```python
from build123d import *

# Parameters (mm, degrees)
F0_W      = 180
F0_H      = 40
F1_DEPTH  = 15
F2_W      = 60
F2_H      = 40
F3_DEPTH  = 120
F4_W      = 41
F4_H      = 40
F5_DEPTH  = 115
F6_R      = 20
F7_R      = 5
F8_W      = 30
F8_H      = 20
F9_DEPTH  = 40
F10_W     = 30
F10_H     = 20
F11_DEPTH = 40
F13_D     = 22
F13_DEPTH = 12
F13_TIP   = 6.6094668093
F15_D     = 22
F15_DEPTH = 12
F15_TIP   = 6.6094668093


with BuildPart() as f1:
    # F0 (on Front) → F1 (new body, symmetric)
    with BuildSketch(Plane.XZ):
        with Locations((0, 6.5696623251)):
            Rectangle(F0_W, F0_H)
    extrude(amount=F1_DEPTH, both=True)

    # F2 (on face) → F3 (join)
    with BuildSketch(Plane.XZ.offset(15)):
        with Locations((0, 6.5696623251)):
            Rectangle(F2_W, F2_H)
    extrude(amount=F3_DEPTH)

    # F4 (on face) → F5 (cut)
    with BuildSketch(Plane.XZ.offset(135)):
        with Locations((0, 6.5696623251)):
            Rectangle(F4_W, F4_H)
    extrude(amount=-F5_DEPTH, mode=Mode.SUBTRACT)

    # F6
    f6_edges = [f1.edges().sort_by_distance(p)[0] for p in [
        (-30, -15, 6.569662),
        (30, -15, 6.569662),
    ]]
    fillet(f6_edges, radius=F6_R)

    # F7
    f7_edges = [f1.edges().sort_by_distance(p)[0] for p in [
        (-20.5, -20, 6.569662),
        (20.5, -20, 6.569662),
        (-20.5, -135, 6.569662),
        (20.5, -135, 6.569662),
    ]]
    fillet(f7_edges, radius=F7_R)

    # F8 (on face) → F9 (cut)
    with BuildSketch(Plane.XY.offset(26.5696623251)):
        with Locations((-70, 0)):
            Rectangle(F8_W, F8_H)
    extrude(amount=-F9_DEPTH, mode=Mode.SUBTRACT)

    # F10 (on face) → F11 (cut)
    with BuildSketch(Plane.XY.offset(26.5696623251)):
        with Locations((70, 0)):
            Rectangle(F10_W, F10_H)
    extrude(amount=-F11_DEPTH, mode=Mode.SUBTRACT)

    # F13
    with Locations(Plane.XZ.offset(15)):
        with Locations((-70, 6.5696623251)):
            Hole(F13_D / 2, depth=F13_DEPTH)
            with Locations((0, 0, -(F13_DEPTH + F13_TIP / 2))):  # 118° drill point
                Cone(0, F13_D / 2, F13_TIP, mode=Mode.SUBTRACT)

    # F15
    with Locations(Plane.XZ.offset(15)):
        with Locations((70, 6.5696623251)):
            Hole(F15_D / 2, depth=F15_DEPTH)
            with Locations((0, 0, -(F15_DEPTH + F15_TIP / 2))):  # 118° drill point
                Cone(0, F15_D / 2, F15_TIP, mode=Mode.SUBTRACT)


solid = f1.part
```
Verification items for the finished model (mm, model axes). A direction names the side the tool comes from. Round coordinates to 2 decimals unless told otherwise and drop trailing zeros. Write each loop counter-clockwise with the first axis right and the second up, starting at its lowest first coordinate (ties: lowest second). Pieces come first, ordered by that corner, then holes. Notation, with made-up numbers: (37, -10.75) - (46, -10.75) arc R16 ccw to (46, 1.25) - close; hole circle Ø11 at (-27, 3). An arc over 180 degrees is marked (long way). Answer as a JSON object with one key per item and string values. Group by question number.
Q1. Thickness scan on line 1 (Z direction, x = -70, y = -12); line 2 (X direction, y = -85.5, z = -10); line 3 (Y direction, x = 61.5, z = -4). Record the ranges inside material, lowest first.
Q2. Section check A-A, the plane y = -108. Enter the section's corners in (x, z), plus the area to 3 significant figures.
Q3. Section check D-D, the plane z = 22. Enter the section's corners in (x, y).
Q4. Go/stop test with flat-tipped pins: pin 1 Ø20 at (x, z) = (-80, 5.5) entering from -Y; pin 2 Ø20 at (y, z) = (-80, 13) entering from +X; pin 3 Ø20 at (y, z) = (-82.5, 15.5) entering from -X; pin 4 Ø6 at (x, y) = (58.5, -8.5) entering from +Z. Record where each tip stops, or that it passes through.
Q5. Section check C-C, the plane x = -70. Enter the section's corners in (y, z).
Q6. Section check B-B, the plane y = 5. Enter the section's corners in (x, z), plus the area to 3 significant figures.
Q7. Tool access check on faces 1 (the flat face through (-79, -15, -2)), 2 (the flat face through (30, -84, 6)), 3 (the flat face through (90, 0, 6)), 4 (the flat face through (-70, 10, 7)), 5 (the cylindrical face through (-22, -133.57, 6.85)). Record the directions out of +Z, -Z, +X, -X, +Y, -Y that give a thin tool (end or side, any length) a straight path to the whole face; none if there is none.
Q8. Mould release check, pull along Y, two halves, no side actions. Record for faces 6 (the flat face through (-55, 0, 7)), 7 (the flat face through (0, -20, 7)), 8 (the flat face through (0, -16, -13.43)), 9 (the flat face through (70, 10, 7)): released by +Y, released by -Y, zero draft, split by the parting line, or undercut.
Found:
{
 "1": {"line 1": "z = -13.43 to -4.43, 17.57 to 26.57", "line 2": "x = -30 to -20.5, 20.5 to 30", "line 3": "y = -15 to -10, 10 to 15"},
 "2": {"outline": "(-30, -13.43) - (-20.5, -13.43) - (-20.5, 26.57) - (-30, 26.57) - close; (20.5, -13.43) - (30, -13.43) - (30, 26.57) - (20.5, 26.57) - close", "area": "760 mm^2"},
 "3": {"outline": "(-90, -15) - (-50, -15) arc R20 cw to (-30, -35) - (-30, -135) - (-25.5, -135) arc R5 ccw to (-20.5, -130) - (-20.5, -25) arc R5 cw to (-15.5, -20) - (15.5, -20) arc R5 cw to (20.5, -25) - (20.5, -130) arc R5 ccw to (25.5, -135) - (30, -135) - (30, -35) arc R20 cw to (50, -15) - (90, -15) - (90, 15) - (-90, 15) - close; hole (-85, -10) - (-55, -10) - (-55, 10) - (-85, 10) - close; hole (55, -10) - (85, -10) - (85, 10) - (55, 10) - close"},
 "4": {"pin 1": "stops at y = -15", "pin 2": "stops at x = 30", "pin 3": "stops at x = -30", "pin 4": "stops at z = 26.57"},
 "5": {"outline": "(-15, -13.43) - (-10, -13.43) - (-10, -4.43) - (-15, -4.43) - close; (-15, 17.57) - (-10, 17.57) - (-10, 26.57) - (-15, 26.57) - close; (10, -13.43) - (15, -13.43) - (15, 26.57) - (10, 26.57) - close"},
 "6": {"outline": "(-90, -13.43) - (-85, -13.43) - (-85, 26.57) - (-90, 26.57) - close; (-55, -13.43) - (55, -13.43) - (55, 26.57) - (-55, 26.57) - close; (85, -13.43) - (90, -13.43) - (90, 26.57) - (85, 26.57) - close", "area": "4,800 mm^2"},
 "7": {"face 1": "+Z, -Z, -X, -Y", "face 2": "+Z, -Z, +X, -Y", "face 3": "+Z, -Z, +X, +Y, -Y", "face 4": "+Z, -Z", "face 5": "+Z, -Z, -Y"},
 "8": {"face 6": "undercut", "face 7": "released by -Y", "face 8": "zero draft", "face 9": "undercut"}
}
